Geometry check sheet. Reference: the model listing, model coordinates, mm. A direction names the side the tool comes from. Give positions to 0.01 mm unless a question says otherwise; leave off trailing zeros. Loops run counter-clockwise (first coordinate to the right, second up) from the corner with the lowest first, then second, coordinate; pieces in that order, holes last. Notation, with made-up numbers: (10, 5) -> (35, 5) arc R17 ccw to (35, 33) -> close; hole circle Ø3 at (68.25, 46.25). An arc over 180 degrees is marked (long way). One line per item, written item: value. Start each with the question number.
(1) Sectioned sample at A-A, the plane z = -236.5. Record the cut outline in (x, y).
(2) Tool access check on faces 4 (the face through (0, -1, -332.5)), 5 (the face through (35.5, -10, 5)). Record the directions out of +Z, -Z, +X, -X, +Y, -Y that give a thin tool (end or side, any length) a straight path to the whole face; none if there is none.
(3) Gauge pin test, flat ends, axial feed: pin 1 Ø4.5 at (y, z) = (-9.5, -200) entering from -X; pin 2 Ø6.5 at (x, z) = (0, -150) entering from -Y. Record the tip position at first contact, or that the pin passes through.
(4) Draft check along X on faces 1 (the face through (0, -1, 332.5)), 2 (the face through (-35.5, -9, 5)), 3 (the face through (37.5, -9, 5)). Enter one of: pulls with the +X half, pulls with the -X half, needs draft (parallel to the pull), parting line crosses it, or undercut.
(5) Sectioned sample at B-B, the plane x = -8.5. Record the cut outline in (y, z), then the cut area to 3 significant figures.
(6) Scan lines: line 1 along X through (y, z) = (-7.5, 297.5); line 2 along Y through (x, z) = (36.9, 100); line 3 along X through (y, z) = (-0.5, 175). Record each from-to range of solid material in increasing order. Write a range as from..to.
from build123d import *

# Parameters (mm, degrees)
SM_BASE_FLANGE_1_DEPTH = 332.5
SKETCH_6_R             = 2.5
CUT_EXTRUDE_1_DEPTH    = 342.183601599
SKETCH_7_R             = 2.5
CUT_EXTRUDE_2_DEPTH    = 10
SKETCH_8_R             = 3.5
CUT_EXTRUDE_3_DEPTH    = 10


# Sheet-metal steps are written as plain solids
with BuildPart() as part:
    # Sketch 1 → Базовая кромка1 (new, symmetric)
    with BuildSketch(Plane.XY):
        with BuildLine():
            Line((-37.5, -15), (-37.5, -4))
            ThreePointArc((-37.5, -4), (-36.328427125, -1.171572875), (-33.5, 0))
            Line((-33.5, 0), (33.5, 0))
            ThreePointArc((33.5, 0), (36.328427125, -1.171572875), (37.5, -4))
            Line((37.5, -4), (37.5, -15))
            Line((37.5, -15), (35.5, -15))
            Line((35.5, -15), (35.5, -4))
            ThreePointArc((35.5, -4), (34.914213562, -2.585786438), (33.5, -2))
            Line((33.5, -2), (-33.5, -2))
            ThreePointArc((-33.5, -2), (-34.914213562, -2.585786438), (-35.5, -4))
            Line((-35.5, -4), (-35.5, -15))
            Line((-35.5, -15), (-37.5, -15))
        make_face()
    extrude(amount=SM_BASE_FLANGE_1_DEPTH, both=True)

    # Эскиз6 → Вырез-Вытянуть1 (cut, through all)
    with BuildSketch(Plane(origin=(37.5, 0, 0), x_dir=(0, 0, -1), z_dir=(1, 0, 0))):
        with Locations((-300, -9.5)):
            Circle(SKETCH_6_R)
        with Locations((-275, -9.5)):
            Circle(SKETCH_6_R)
        with Locations((-250, -9.5)):
            Circle(SKETCH_6_R)
        with Locations((-225, -9.5)):
            Circle(SKETCH_6_R)
        with Locations((-200, -9.5)):
            Circle(SKETCH_6_R)
        with Locations((-175, -9.5)):
            Circle(SKETCH_6_R)
        with Locations((-150, -9.5)):
            Circle(SKETCH_6_R)
        with Locations((-125, -9.5)):
            Circle(SKETCH_6_R)
        with Locations((-100, -9.5)):
            Circle(SKETCH_6_R)
        with Locations((-75, -9.5)):
            Circle(SKETCH_6_R)
        with Locations((-50, -9.5)):
            Circle(SKETCH_6_R)
        with Locations((-25, -9.5)):
            Circle(SKETCH_6_R)
        with Locations((0, -9.5)):
            Circle(SKETCH_6_R)
        with Locations((25, -9.5)):
            Circle(SKETCH_6_R)
        with Locations((50, -9.5)):
            Circle(SKETCH_6_R)
        with Locations((75, -9.5)):
            Circle(SKETCH_6_R)
        with Locations((100, -9.5)):
            Circle(SKETCH_6_R)
        with Locations((125, -9.5)):
            Circle(SKETCH_6_R)
        with Locations((150, -9.5)):
            Circle(SKETCH_6_R)
        with Locations((175, -9.5)):
            Circle(SKETCH_6_R)
        with Locations((200, -9.5)):
            Circle(SKETCH_6_R)
        with Locations((225, -9.5)):
            Circle(SKETCH_6_R)
        with Locations((250, -9.5)):
            Circle(SKETCH_6_R)
        with Locations((275, -9.5)):
            Circle(SKETCH_6_R)
        with Locations((300, -9.5)):
            Circle(SKETCH_6_R)
        with Locations((325, -9.5)):
            Circle(SKETCH_6_R)
        with Locations((350, -9.5)):
            Circle(SKETCH_6_R)
        with Locations((375, -9.5)):
            Circle(SKETCH_6_R)
        with Locations((400, -9.5)):
            Circle(SKETCH_6_R)
        with Locations((425, -9.5)):
            Circle(SKETCH_6_R)
        with Locations((450, -9.5)):
            Circle(SKETCH_6_R)
        with Locations((475, -9.5)):
            Circle(SKETCH_6_R)
        with Locations((500, -9.5)):
            Circle(SKETCH_6_R)
        with Locations((525, -9.5)):
            Circle(SKETCH_6_R)
        with Locations((550, -9.5)):
            Circle(SKETCH_6_R)
        with Locations((575, -9.5)):
            Circle(SKETCH_6_R)
    extrude(amount=-CUT_EXTRUDE_1_DEPTH, mode=Mode.SUBTRACT)

    # Эскиз7 → Вырез-Вытянуть2 (cut)
    with BuildSketch(Plane(origin=(0, 0, 0), x_dir=(1, 0, 0), z_dir=(0, 1, 0))):
        with Locations(Location((0, 300, 0), (0, 0, 180))):
            Circle(SKETCH_7_R)
        with Locations(Location((0, 275, 0), (0, 0, 180))):
            Circle(SKETCH_7_R)
        with Locations(Location((0, 250, 0), (0, 0, 180))):
            Circle(SKETCH_7_R)
        with Locations(Location((0, 225, 0), (0, 0, 180))):
            Circle(SKETCH_7_R)
        with Locations(Location((0, 200, 0), (0, 0, 180))):
            Circle(SKETCH_7_R)
        with Locations(Location((0, 175, 0), (0, 0, 180))):
            Circle(SKETCH_7_R)
        with Locations(Location((0, 150, 0), (0, 0, 180))):
            Circle(SKETCH_7_R)
        with Locations(Location((0, 125, 0), (0, 0, 180))):
            Circle(SKETCH_7_R)
        with Locations(Location((0, 100, 0), (0, 0, 180))):
            Circle(SKETCH_7_R)
        with Locations(Location((0, 75, 0), (0, 0, 180))):
            Circle(SKETCH_7_R)
        with Locations(Location((0, 50, 0), (0, 0, 180))):
            Circle(SKETCH_7_R)
        with Locations(Location((0, 25, 0), (0, 0, 180))):
            Circle(SKETCH_7_R)
        with Locations(Location((0, 0, 0), (0, 0, 180))):
            Circle(SKETCH_7_R)
        with Locations(Location((0, -25, 0), (0, 0, 180))):
            Circle(SKETCH_7_R)
        with Locations(Location((0, -50, 0), (0, 0, 180))):
            Circle(SKETCH_7_R)
        with Locations(Location((0, -75, 0), (0, 0, 180))):
            Circle(SKETCH_7_R)
        with Locations(Location((0, -100, 0), (0, 0, 180))):
            Circle(SKETCH_7_R)
        with Locations(Location((0, -125, 0), (0, 0, 180))):
            Circle(SKETCH_7_R)
        with Locations(Location((0, -150, 0), (0, 0, 180))):
            Circle(SKETCH_7_R)
        with Locations(Location((0, -175, 0), (0, 0, 180))):
            Circle(SKETCH_7_R)
        with Locations(Location((0, -200, 0), (0, 0, 180))):
            Circle(SKETCH_7_R)
        with Locations(Location((0, -225, 0), (0, 0, 180))):
            Circle(SKETCH_7_R)
        with Locations(Location((0, -250, 0), (0, 0, 180))):
            Circle(SKETCH_7_R)
        with Locations(Location((0, -275, 0), (0, 0, 180))):
            Circle(SKETCH_7_R)
        with Locations(Location((0, -300, 0), (0, 0, 180))):
            Circle(SKETCH_7_R)
    extrude(amount=-CUT_EXTRUDE_2_DEPTH, mode=Mode.SUBTRACT)

    # Эскиз8 → Вырез-Вытянуть3 (cut)
    with BuildSketch(Plane(origin=(0, 0, 0), x_dir=(1, 0, 0), z_dir=(0, 1, 0))):
        with Locations(Location((25, 325, 0), (0, 0, 180))):
            Circle(SKETCH_8_R)
        with Locations(Location((-25, 325, 0), (0, 0, 180))):
            Circle(SKETCH_8_R)
        with Locations((-25, -325)):
            Circle(SKETCH_8_R)
        with Locations((25, -325)):
            Circle(SKETCH_8_R)
    extrude(amount=-CUT_EXTRUDE_3_DEPTH, mode=Mode.SUBTRACT)


solid = part.part
Calculated:
1. outline: (-37.5, -15) -> (-35.5, -15) -> (-35.5, -4) arc R2 cw to (-33.5, -2) -> (33.5, -2) arc R2 cw to (35.5, -4) -> (35.5, -15) -> (37.5, -15) -> (37.5, -4) arc R4 ccw to (33.5, 0) -> (-33.5, 0) arc R4 ccw to (-37.5, -4) -> close
2. face 4: -Z, +X, -X, +Y, -Y
2. face 5: +Z, -Z, -Y
3. pin 1: passes through
3. pin 2: stops at y = -2
4. face 1: needs draft
4. face 2: undercut
4. face 3: pulls with the +X half
5. outline: (-2, -332.5) -> (0, -332.5) -> (0, 332.5) -> (-2, 332.5) -> close
5. area: 1,330 mm2
6. line 1: x = -37.5..-35.5, 35.5..37.5
6. line 2: y = -15..-12, -7..-1.89
6. line 3: x = -35.44..-2.5, 2.5..35.44
